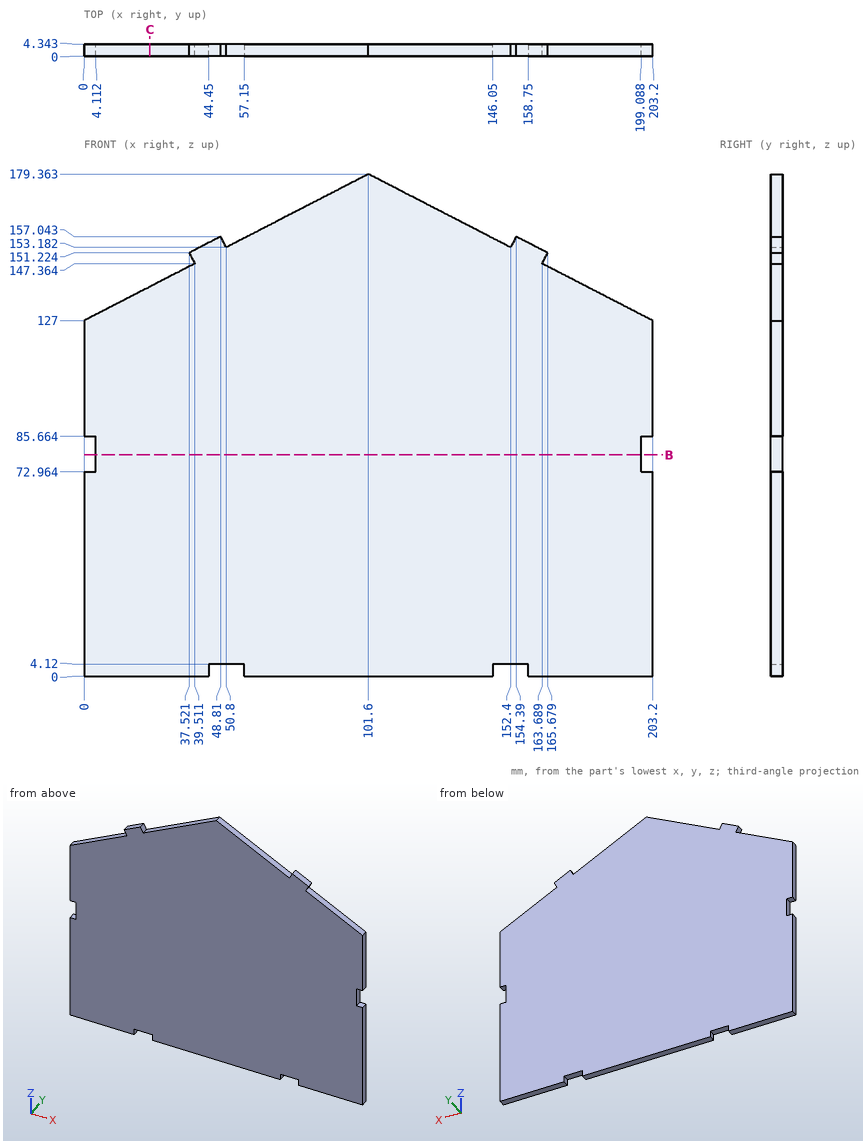
Design review of the part shown in the three views and the two pictorial views. Dimensions are in mm from the part's minimum x, y and z. Give positions to 0.01 mm unless a question says otherwise; leave off trailing zeros. Write each loop counter-clockwise with the first axis right and the second up, starting at its lowest first coordinate (ties: lowest second). Pieces come first, ordered by that corner, then holes. Notation, with made-up numbers: M -26,74 L 27,74 A16 ccw 27,79 Z; hole C 10,3 d7. An arc over 180 degrees is marked long. Return JSON: item names as keys, results as strings. Group by question number.
Item 1: Clearance check with flat-ended pins moving along their axes: pin 1 Ø2 at (y, z) = (0.5, 48.5) entering from -X; pin 2 Ø1.2 at (x, y) = (2.5, 2) entering from +Z; pin 3 Ø2 at (x, y) = (202, 1.5) entering from +Z (1 decimal); pin 4 Ø2 at (y, z) = (2, 78.5) entering from +X. State where each tip first meets the part, or that it passes through.
Item 2: Wall thickness on line 1 along X through (y, z) = (1.05, 83.5); line 2 along Z through (x, y) = (27.5, 2.15) (1 decimal); line 3 along Z through (x, y) = (11.5, 2.45): over which ranges is each line inside the solid? List them lowest first.
Item 3: Take a section at B-B (z = 79). Give the boundary of the cut face in (x, y).
Item 4: Take a section at C-C (x = 23.5). Give the boundary of the cut face in (y, z).
Return value:
{
 "1": {"pin 1": "stops at x = 0", "pin 2": "stops at z = 128.6", "pin 3": "stops at z = 128.1", "pin 4": "stops at x = 199.09"},
 "2": {"line 1": "x = 4.11 to 199.09", "line 2": "z = 0 to 141.2", "line 3": "z = 0 to 132.93"},
 "3": {"outline": "M 4.11,0 L 199.09,0 L 199.09,4.34 L 4.11,4.34 Z"},
 "4": {"outline": "M 0,0 L 4.34,0 L 4.34,139.11 L 0,139.11 Z"}
}
